For this review, take the finished solid that the model builds, in its own axes (mm). A direction names the side the tool comes from. Give positions to 0.01 mm unless a question says otherwise; leave off trailing zeros. Write each loop counter-clockwise with the first axis right and the second up, starting at its lowest first coordinate (ties: lowest second). Pieces come first, ordered by that corner, then holes.
1) For P1, Ø1.5, axis at y = 19, z = 5.5, coming from the -X side; P2, Ø10, axis at x = -27, y = 26, coming from the -Z side; P3, Ø10.5, axis at y = -24.5, z = 35.5, coming from the +X side; P4, Ø4, axis at y = 27, z = 6, coming from the +X side, all flat-tipped, find the tip position at first contact; note any pin that passes through.
2) Wall thickness on line 1 along Y through (x, z) = (15, 11.5); line 2 along Y through (x, z) = (-21, 17); line 3 along X through (y, z) = (-19.5, 22.5): over which ranges is each line inside the solid? List them lowest first.
3) We need section A-A on y = 0. Give the boundary of the cut face in (x, z), and give its area (3 significant figures).
4) Machinability: for faces 5 (the face through (20.567, 19.152, 24.883)), 6 (the face through (-3.367, -25.307, 25.35)), 7 (the face through (8.235, 26.87, 24.883)), 8 (the face through (7.629, -28.528, 25.35)), which of the approach directions +Z, -Z, +X, -X, +Y, -Y give a long, thin tool a straight path to every point of the face, cutting with its end or side? Answer none if there is none.
5) Draft analysis for pull direction Y (two halves, no side actions). For faces 1 (the face through (-14.909, -23.823, 24.883)), 2 (the face through (-20.87, 20.89, 25.35)), 3 (the face through (29.53, -0.01, 25.35)), 4 (the face through (19.152, -20.567, 24.883)), state which applies: pulls with the +Y half, pulls with the -Y half, needs draft (parallel to the pull), parting line crosses it, or undercut.
from build123d import *

# Parameters (mm, degrees)
SKETCH1_R           = 30
BOSS_EXTRUDE6_DEPTH = 50
BOSS_EXTRUDE6_TAPER = 10
SKETCH5_R           = 28
CUT_EXTRUDE1_DEPTH  = 50
CUT_EXTRUDE1_TAPER  = 10
SKETCH6_R           = 21.183650965
BOSS_EXTRUDE7_DEPTH = 5
BOSS_EXTRUDE8_DEPTH = 1
CIRPATTERN2_COUNT   = 24


with BuildPart() as part:
    # Sketch1 → Boss-Extrude6 (new body)
    with BuildSketch(Plane.XY):
        Circle(SKETCH1_R)
    extrude(amount=BOSS_EXTRUDE6_DEPTH, taper=BOSS_EXTRUDE6_TAPER)

    # Sketch5 → Cut-Extrude1 (cut)
    with BuildSketch(Plane.XY):
        Circle(SKETCH5_R)
    extrude(amount=CUT_EXTRUDE1_DEPTH, taper=CUT_EXTRUDE1_TAPER, mode=Mode.SUBTRACT)

    # Sketch6 → Boss-Extrude7 (add)
    with BuildSketch(Plane.XY.offset(50)):
        Circle(SKETCH6_R)
    extrude(amount=-BOSS_EXTRUDE7_DEPTH)

    # Sketch7 → Boss-Extrude8 (add, symmetric)
    with BuildSketch(Plane(origin=(0, 0, 0), x_dir=(0, 0, -1), z_dir=(1, 0, 0))):
        Polygon((0, 28), (-50, 19.183650965), (-50, 25.183650965), (0, 34), align=None)
    boss_extrude8 = extrude(amount=BOSS_EXTRUDE8_DEPTH, both=True)

    # CirPattern2: Boss-Extrude8 ×24 about axis
    cirpattern2_axis = Axis((0, 0, 0), (0, 0, 1))
    for i in range(1, CIRPATTERN2_COUNT):
        add(boss_extrude8.rotate(cirpattern2_axis, i * 360 / CIRPATTERN2_COUNT))


solid = part.part
Results list:
1. P1: stops at x = -22.6
1. P2: stops at z = 0
1. P3: stops at x = 20.14
1. P4: stops at x = 17.47
2. line 1: y = -27.98 to -23.98, -23.61 to -21.2, 21.2 to 23.61, 23.98 to 27.98
2. line 2: y = -22.41 to -19.59, -16.97 to -13.57, 13.57 to 16.97, 19.59 to 22.41
2. line 3: x = -20.91 to -18.09, -17.25 to -14.05, 14.05 to 17.25, 18.09 to 20.91
3. outline: (-34, 0) - (-28, 0) - (-20.07, 45) - (20.07, 45) - (28, 0) - (34, 0) - (25.18, 50) - (-25.18, 50) - close
3. area: 796 mm2
4. face 5: +Z, +X
4. face 6: +Z, -Y
4. face 7: +Z
4. face 8: +Z, +X, -Y
5. face 1: undercut
5. face 2: pulls with the +Y half
5. face 3: needs draft
5. face 4: pulls with the -Y half
